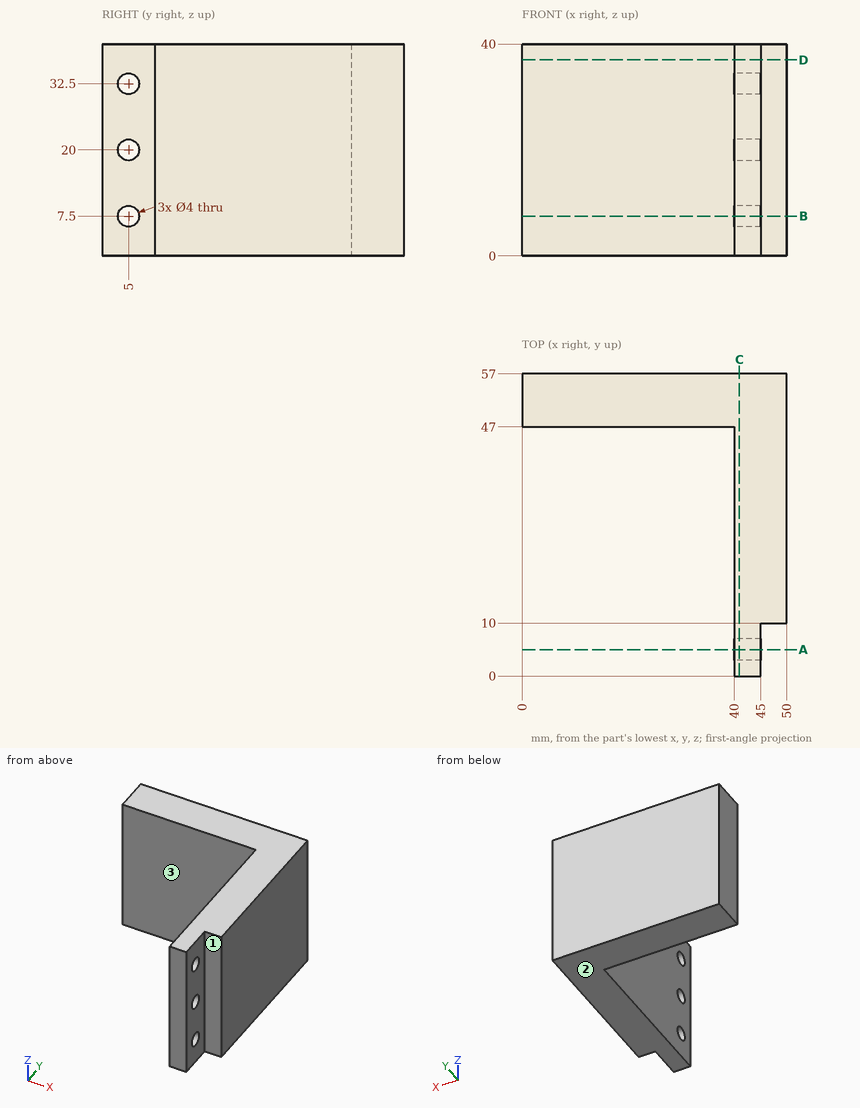
Here's the drawing with two shaded views (mm, measured from the low corner). I have some questions. A direction names the side the tool comes from. Give positions to 0.01 mm unless a question says otherwise; leave off trailing zeros. Order: outer loops, then holes, each group sorted by start corner. A loop starts at its lowest first (then second) coordinate and runs counter-clockwise, first axis right, second up. Notation, with made-up numbers: (-7, -23) -> (12, -23) arc R31 ccw to (12, 15) -> close; hole circle Ø6 at (35.5, 30.5). An arc over 180 degrees is marked (long way). One line per item, written item: value. Start each with the question number.
1. I need wall thicknesses on probe 1 along Y at (x, z) = (41.25, 7.5); probe 2 along X at (y, z) = (25.5, 21); probe 3 along Y at (x, z) = (5, 33). Which ranges of each line are inside material? Lowest first, please. Write a range as from..to.
2. Imagine slicing it at B-B, the plane z = 7.5. List the corners of the cut face in (x, y) for me.
3. Imagine slicing it at C-C, the plane x = 41. List the corners of the cut face in (y, z) for me, plus the area to 3 significant figures.
4. Imagine slicing it at A-A, the plane y = 5. List the corners of the cut face in (x, z) for me, plus the area to 3 significant figures.
5. Will these pins go through, and if not, where does the flat tip stop? pin 1 Ø1.5 at (x, z) = (47.5, 17.5) entering from -Y; pin 2 Ø3 at (y, z) = (3, 16) entering from +X; pin 3 Ø3.5 at (y, z) = (5, 7.5) entering from +X; pin 4 Ø6.5 at (y, z) = (5, 20) entering from -X.
6. For the marked faces 1, 2 and 3, which set-ups out of +Z, -Z, +X, -X, +Y, -Y let a thin tool reach every point of the face, with its end or its side?
7. Imagine slicing it at D-D, the plane z = 37. List the corners of the cut face in (x, y) for me.
Values follow:
1. probe 1: y = 0..3, 7..57
1. probe 2: x = 40..50
1. probe 3: y = 47..57
2. outline: (0, 47) -> (40, 47) -> (40, 7) -> (45, 7) -> (45, 10) -> (50, 10) -> (50, 57) -> (0, 57) -> close; (40, 0) -> (45, 0) -> (45, 3) -> (40, 3) -> close
3. outline: (0, 0) -> (57, 0) -> (57, 40) -> (0, 40) -> close; hole circle Ø4 at (5, 7.5); hole circle Ø4 at (5, 20); hole circle Ø4 at (5, 32.5)
3. area: 2,240 mm2
4. outline: (40, 0) -> (45, 0) -> (45, 5.5) -> (40, 5.5) -> close; (40, 9.5) -> (45, 9.5) -> (45, 18) -> (40, 18) -> close; (40, 22) -> (45, 22) -> (45, 30.5) -> (40, 30.5) -> close; (40, 34.5) -> (45, 34.5) -> (45, 40) -> (40, 40) -> close
4. area: 140 mm2
5. pin 1: stops at y = 10
5. pin 2: stops at x = 45
5. pin 3: passes through
5. pin 4: stops at x = 40
6. face 1: +Z, -Z, +X, -Y
6. face 2: -Z, +X, -X, +Y, -Y
6. face 3: +Z, -Z, -X, -Y
7. outline: (0, 47) -> (40, 47) -> (40, 0) -> (45, 0) -> (45, 10) -> (50, 10) -> (50, 57) -> (0, 57) -> close
